The model under review builds one solid part; all positions refer to its coordinate system, in mm. A direction names the side the tool comes from. Coordinates: 2 decimals unless noted, no trailing zeros. Order: outer loops, then holes, each group sorted by start corner. A loop starts at its lowest first (then second) coordinate and runs counter-clockwise, first axis right, second up. Notation, with made-up numbers: (-6, 88) - (34, 88) arc R13 ccw to (34, 111) - close; hole circle Ø1 at (39, 37). An arc over 180 degrees is marked (long way). Answer in a Markdown table with one row per item.
```python
from build123d import *

# Parameters (mm, degrees)
SKETCH1_W                                      = 12
SKETCH1_H                                      = 30.5
SKETCH1_R                                      = 1.383995923
SKETCH1_R_2                                    = 1.420525084
BOSS_EXTRUDE1_DEPTH                            = 3
CSK_FOR_M3_FLAT_HEAD_MACHINE_SCREW1_AT_2_COUNT = 2
CSK_FOR_M3_FLAT_HEAD_MACHINE_SCREW1_AT_2_PITCH = 15


with BuildPart() as part:
    # Sketch1 → Boss-Extrude1 (new body)
    with BuildSketch(Plane.XY):
        Polygon((-6, 12.25), (-6, 15.25), (-38, 15.25), (-38, -15.25), (-6, -15.25), (-6, -8.75), (-13, -8.75), (-13, 12.25), align=None)
        Rectangle(SKETCH1_W, SKETCH1_H)
        with Locations((-0.2, 7.25)):
            Circle(SKETCH1_R, mode=Mode.SUBTRACT)
        with Locations((-0.2, -7.75)):
            Circle(SKETCH1_R_2, mode=Mode.SUBTRACT)
    extrude(amount=BOSS_EXTRUDE1_DEPTH)

    # Sketch4 → CSK for M3 Flat Head Machine Screw1 (revolve, cut)
    with BuildSketch(Plane(origin=(-0.2, 7.25, 3), x_dir=(0, -1, 0), z_dir=(1, 0, 0))):
        Polygon((0, 0), (0, 3), (1.7, 3), (1.7, 1.45), (3.15, 0), align=None)
    csk_for_m3_flat_head_machine_screw1 = revolve(axis=Axis((-0.2, 7.25, 9.35), (0, 0, -1)), mode=Mode.SUBTRACT)

    # CSK for M3 Flat Head Machine Screw1 at 2: CSK for M3 Flat Head Machine Screw1 ×2
    with Locations(*[(0, -i * CSK_FOR_M3_FLAT_HEAD_MACHINE_SCREW1_AT_2_PITCH, 0) for i in range(1, CSK_FOR_M3_FLAT_HEAD_MACHINE_SCREW1_AT_2_COUNT)]):
        add(csk_for_m3_flat_head_machine_screw1, mode=Mode.SUBTRACT)


solid = part.part
```
Item 1: We need section B-B, the plane z = 2.4. Write out the cut boundary in (x, y).
Check values:
| item | result |
|---|---|
| outline | (-38, -15.25) - (6, -15.25) - (6, 15.25) - (-38, 15.25) - close; hole (-13, -8.75) - (-6, -8.75) - (-6, 12.25) - (-13, 12.25) - close; hole circle Ø5.1 at (-0.2, -7.75); hole circle Ø5.1 at (-0.2, 7.25) |
Item 2: To check wall thickness, follow line 1 (Y direction, x = -0.2, z = 0.45); line 2 (Y direction, x = -8, z = 0.25); line 3 (X direction, y = 7.25, z = 1). State the ranges of each line that lie inside material, in increasing order. Write a range as from..to.
Check values:
| item | result |
|---|---|
| line 1 | -15.25..-9.45, -6.05..5.55, 8.95..15.25 |
| line 2 | -15.25..-8.75, 12.25..15.25 |
| line 3 | -38..-13, -6..-1.9, 1.5..6 |
Item 3: We need section D-D, the plane y = -3. Write out the cut boundary in (x, z).
Check values:
| item | result |
|---|---|
| outline | (-38, 0) - (-13, 0) - (-13, 3) - (-38, 3) - close; (-6, 0) - (6, 0) - (6, 3) - (-6, 3) - close |
Item 4: We need section C-C, the plane x = -0.2. Write out the cut boundary in (y, z), then the cut area to 3 significant figures.
Check values:
| item | result |
|---|---|
| outline | (-15.25, 0) - (-9.45, 0) - (-9.45, 1.55) - (-10.9, 3) - (-15.25, 3) - close; (-6.05, 0) - (5.55, 0) - (5.55, 1.55) - (4.1, 3) - (-4.6, 3) - (-6.05, 1.55) - close; (8.95, 0) - (15.25, 0) - (15.25, 3) - (10.4, 3) - (8.95, 1.55) - close |
| area | 66.9 mm^2 |
Item 5: We need section A-A, the plane y = -7.75. Write out the cut boundary in (x, z).
Check values:
| item | result |
|---|---|
| outline | (-38, 0) - (-13, 0) - (-13, 3) - (-38, 3) - close; (-6, 0) - (-1.9, 0) - (-1.9, 1.55) - (-3.35, 3) - (-6, 3) - close; (1.5, 0) - (6, 0) - (6, 3) - (2.95, 3) - (1.5, 1.55) - close |
Item 6: Clearance check with a flat-ended pin moving along its axis: pin 1 Ø2 at (x, y) = (-0.2, 7.25) entering from +Z. State where the tip first meets the part, or that it passes through.
Check values:
| item | result |
|---|---|
| pin 1 | through |
Item 7: Tool access review of faces 4 (the face through (-16, -15.25, 1)), 5 (the face through (-9, -8.75, 1)): name each direction out of +Z, -Z, +X, -X, +Y, -Y from which nothing blocks a thin tool from reaching the whole face with its end or side.
Check values:
| item | result |
|---|---|
| face 4 | +Z, -Z, +X, -X, -Y |
| face 5 | +Z, -Z |
Item 8: Mouldability with a two-part tool opening along X and no side actions: class faces 1 (the face through (-38, 0, 1)), 2 (the face through (-0.27, 8.95, 0.79)), 3 (the face through (-16, 0, 0)) as +X half, -X half, draft (parallel to the pull), parting line (faces both ways), or undercut.
Check values:
| item | result |
|---|---|
| face 1 | -X half |
| face 2 | undercut |
| face 3 | draft |
